Check sheet for the drawn part. Datum: minimum x, y, z corner. Units: mm. Round coordinates to 2 decimals unless told otherwise and drop trailing zeros. Loops run counter-clockwise (first coordinate to the right, second up) from the corner with the lowest first, then second, coordinate; pieces in that order, holes last.
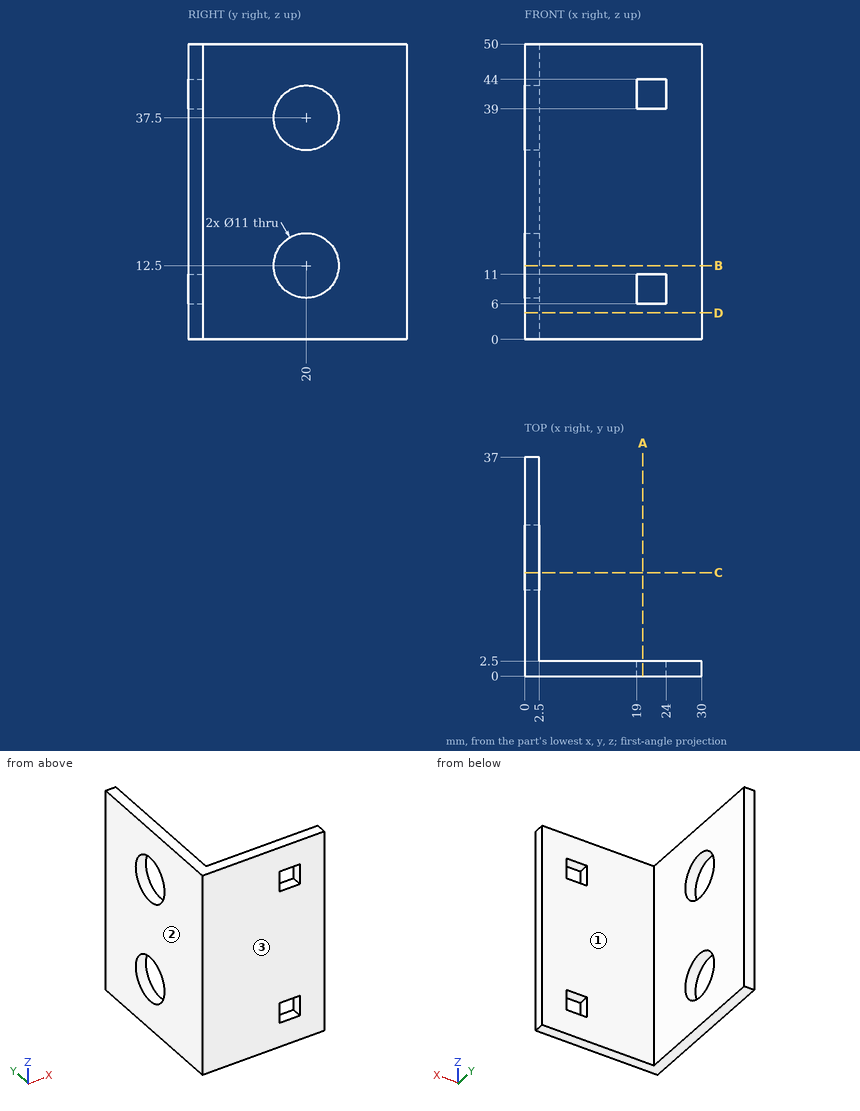
1) Sectioned sample at B-B, the plane z = 12.5. Record the cut outline in (x, y), then the cut area to 3 significant figures.
Report:
outline: (0, 0) - (30, 0) - (30, 2.5) - (2.5, 2.5) - (2.5, 14.5) - (0, 14.5) - close; (0, 25.5) - (2.5, 25.5) - (2.5, 37) - (0, 37) - close
area: 134 mm2
2) Sectioned sample at D-D, the plane z = 4.5. Record the cut outline in (x, y), then the cut area to 3 significant figures.
Report:
outline: (0, 0) - (30, 0) - (30, 2.5) - (2.5, 2.5) - (2.5, 37) - (0, 37) - close
area: 161 mm2
3) Mould release check, pull along Y, two halves, no side actions. Record for the marked faces 1, 2 and 3: +Y half, -Y half, draft (parallel to the pull), parting line (faces both ways), or undercut.
Report:
face 1: +Y half
face 2: draft
face 3: -Y half
4) Sectioned sample at C-C, the plane y = 17.5. Record the cut outline in (x, z).
Report:
outline: (0, 0) - (2.5, 0) - (2.5, 7.6) - (0, 7.6) - close; (0, 17.4) - (2.5, 17.4) - (2.5, 32.6) - (0, 32.6) - close; (0, 42.4) - (2.5, 42.4) - (2.5, 50) - (0, 50) - close
5) Gauge pin test, flat ends, axial feed: pin 1 (5 mm diameter, centred on y = 12, z = 30.5, fed in from +X); pin 2 (4 mm diameter, centred on x = 8.5, z = 42, fed in from +Y). Record the tip position at first contact, or that the pin passes through.
Report:
pin 1: stops at x = 2.5
pin 2: stops at y = 2.5
6) Sectioned sample at A-A, the plane x = 20. Record the cut outline in (y, z), then the cut area to 3 significant figures.
Report:
outline: (0, 0) - (2.5, 0) - (2.5, 6) - (0, 6) - close; (0, 11) - (2.5, 11) - (2.5, 39) - (0, 39) - close; (0, 44) - (2.5, 44) - (2.5, 50) - (0, 50) - close
area: 100 mm2
7) Scan lines: line 1 along Y through (x, z) = (1, 12.5); line 2 along X through (y, z) = (10, 28.5). Record each from-to range of solid material in increasing order.
Report:
line 1: y = 0 to 14.5, 25.5 to 37
line 2: x = 0 to 2.5
